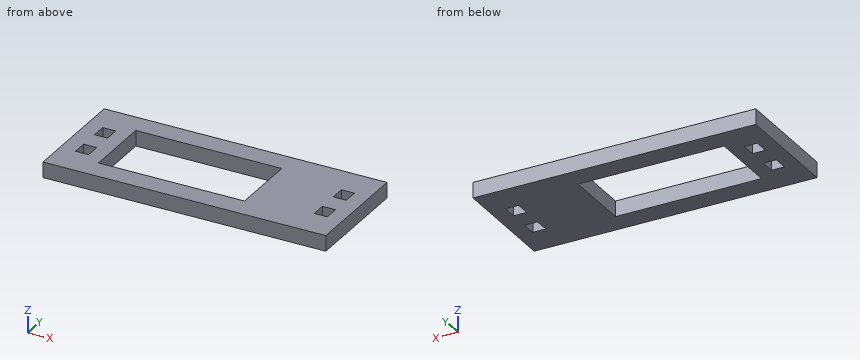
```python
from build123d import *

# Parameters (mm, degrees)
SKETCH1_W           = 115.57
SKETCH1_H           = 45.72
BOSS_EXTRUDE1_DEPTH = 6.35
SKETCH2_W           = 59.69
SKETCH2_H           = 27.94
CUT_EXTRUDE1_DEPTH  = 7.35
SKETCH3_W           = 5.334
SKETCH3_H           = 6.096
CUT_EXTRUDE2_DEPTH  = 7.35


with BuildPart() as part:
    # Sketch1 → Boss-Extrude1 (new body)
    with BuildSketch(Plane.XY):
        Rectangle(SKETCH1_W, SKETCH1_H)
    extrude(amount=BOSS_EXTRUDE1_DEPTH)

    # Sketch2 → Cut-Extrude1 (cut, through all)
    with BuildSketch(Plane.XY.offset(6.35)):
        with Locations((-10.16, 0)):
            Rectangle(SKETCH2_W, SKETCH2_H)
    extrude(amount=-CUT_EXTRUDE1_DEPTH, mode=Mode.SUBTRACT)

    # Sketch3 → Cut-Extrude2 (cut, through all)
    with BuildSketch(Plane.XY.offset(6.35)):
        with Locations((-48.768, 7.112)):
            Rectangle(SKETCH3_W, SKETCH3_H)
        with Locations((-48.768, -7.112)):
            Rectangle(SKETCH3_W, SKETCH3_H)
        with Locations((48.768, -7.112)):
            Rectangle(SKETCH3_W, SKETCH3_H)
        with Locations((48.768, 7.112)):
            Rectangle(SKETCH3_W, SKETCH3_H)
    extrude(amount=-CUT_EXTRUDE2_DEPTH, mode=Mode.SUBTRACT)


solid = part.part
```
Design review of the part built by this model. Coordinates are the model's own, in mm. Round coordinates to 2 decimals unless told otherwise and drop trailing zeros. Order: outer loops, then holes, each group sorted by start corner. A loop starts at its lowest first (then second) coordinate and runs counter-clockwise, first axis right, second up. Notation, with made-up numbers: (37, 28) - (64, 28) arc R13 ccw to (64, 53) - close; hole circle Ø11 at (80, 10). An arc over 180 degrees is marked (long way). Return JSON: item names as keys, results as strings.
Q1. Consider section A-A on x = -9.5. Write out the cut boundary in (y, z).
Computed values:
{"outline": "(-22.86, 0) - (-13.97, 0) - (-13.97, 6.35) - (-22.86, 6.35) - close; (13.97, 0) - (22.86, 0) - (22.86, 6.35) - (13.97, 6.35) - close"}
Q2. Wall thickness on L1, parallel to X at y = -5, z = 2.75 (3 decimals); L2, parallel to Y at x = 14.5, z = 3.75; L3, parallel to X at y = -3, z = 4.5 (3 decimals): over which ranges is each line inside the solid? List them lowest first. Write a range as [from, to].
Computed values:
{"L1": "x = [-57.785, -51.435], [-46.101, -40.005], [19.685, 46.101], [51.435, 57.785]", "L2": "y = [-22.86, -13.97], [13.97, 22.86]", "L3": "x = [-57.785, -40.005], [19.685, 57.785]"}
Q3. Consider section B-B on y = -0.5. Write out the cut boundary in (x, z) (3 decimals).
Computed values:
{"outline": "(-57.785, 0) - (-40.005, 0) - (-40.005, 6.35) - (-57.785, 6.35) - close; (19.685, 0) - (57.785, 0) - (57.785, 6.35) - (19.685, 6.35) - close"}
Q4. Consider section C-C on z = 3. Write out the cut boundary in (x, y) (3 decimals), plus the area to 3 significant figures.
Computed values:
{"outline": "(-57.785, -22.86) - (57.785, -22.86) - (57.785, 22.86) - (-57.785, 22.86) - close; hole (-51.435, -10.16) - (-46.101, -10.16) - (-46.101, -4.064) - (-51.435, -4.064) - close; hole (-51.435, 4.064) - (-46.101, 4.064) - (-46.101, 10.16) - (-51.435, 10.16) - close; hole (-40.005, -13.97) - (19.685, -13.97) - (19.685, 13.97) - (-40.005, 13.97) - close; hole (46.101, -10.16) - (51.435, -10.16) - (51.435, -4.064) - (46.101, -4.064) - close; hole (46.101, 4.064) - (51.435, 4.064) - (51.435, 10.16) - (46.101, 10.16) - close", "area": "3,490 mm2"}
Q5. Consider section D-D on y = 8. Write out the cut boundary in (x, z) (3 decimals), plus the area to 3 significant figures.
Computed values:
{"outline": "(-57.785, 0) - (-51.435, 0) - (-51.435, 6.35) - (-57.785, 6.35) - close; (-46.101, 0) - (-40.005, 0) - (-40.005, 6.35) - (-46.101, 6.35) - close; (19.685, 0) - (46.101, 0) - (46.101, 6.35) - (19.685, 6.35) - close; (51.435, 0) - (57.785, 0) - (57.785, 6.35) - (51.435, 6.35) - close", "area": "287 mm2"}
Q6. For pin 1 Ø10 at (x, y) = (-17, 4.5) entering from +Z, flat-tipped, find the tip position at first contact; note if it passes through.
Computed values:
{"pin 1": "passes through"}
